The listing builds one solid part. Answer for the finished solid, in the listing's coordinates (mm). A direction names the side the tool comes from. Round coordinates to 2 decimals unless told otherwise and drop trailing zeros. Order: outer loops, then holes, each group sorted by start corner. A loop starts at its lowest first (then second) coordinate and runs counter-clockwise, first axis right, second up. Notation, with made-up numbers: (-38.75, 38.5) - (-17.75, 38.5) arc R25 ccw to (-17.75, 57.5) - close; hole circle Ø3 at (75.5, 32). An arc over 180 degrees is marked (long way). One line per item, written item: value. Start each with the question number.
1. Section A-A, the plane x = -40 is taken. Give the vertices of the cut face in (y, z), then the cut area to 3 significant figures.
2. A tool of negligible diameter and unlimited length cuts with its end or side. For faces 1 (the flat face through (-18, 0, -4.318)), 2 (the cylindrical face through (-5.586, 5.253, -2.129)), 3 (the cylindrical face through (-41.083, 13.974, 15.083)), from which of +Z, -Z, +X, -X, +Y, -Y can it reach the whole face along a straight path? Write none if from no direction.
3. Section B-B, the plane y = -26 is taken. Give the vertices of the cut face in (x, z).
4. Flat-ended cylindrical pins translate along their axes: P1, Ø3, axis at x = -9.5, y = 11, coming from the +Z side; P2, Ø12, axis at x = -41.5, z = 6, coming from the -Y side; P3, Ø2, axis at x = -35.5, z = 10, coming from the +Y side. Find the tip coordinate at first contact, or state that the pin passes through.
5. Section C-C, the plane z = 9.5 is taken. Give the vertices of the cut face in (x, y), then the cut area to 3 significant figures.
6. Section D-D, the plane x = -20.5 is taken. Give the vertices of the cut face in (y, z), then the cut area to 3 significant figures.
7. Straight lines are drawn through the part: line 1 (Z direction, x = -33, y = 7); line 2 (Z direction, x = -52, y = -16.5); line 3 (Y direction, x = -19, z = -3). For each, find the intervals that lie inside material, in ascending order.
from build123d import *

# Parameters (mm, degrees)
F0_R     = 43.938872
F1_DEPTH = 12.954
F2_R     = 13.186842
F3_DEPTH = 4.318
F4_R     = 13.716315
F5_DEPTH = 4.318


with BuildPart() as f1:
    # F0 (on Top) → F1 (new body)
    with BuildSketch(Plane.XY):
        with Locations((-21.176565, 11.984369)):
            Circle(F0_R)
    extrude(amount=F1_DEPTH)

    # F2 (on face) → F3 (join)
    with BuildSketch(Plane.XY.offset(12.954)):
        with Locations((-27.908787, 13.394361)):
            Circle(F2_R)
    extrude(amount=F3_DEPTH)

    # F4 (on face) → F5 (join)
    with BuildSketch(Plane(origin=(0, 0, 0), x_dir=(1, 0, 0), z_dir=(0, 0, -1))):
        with Locations((-18.256115, 0)):
            Circle(F4_R)
    extrude(amount=F5_DEPTH)


solid = f1.part
Answer list:
1. outline: (-27.72, 0) - (51.69, 0) - (51.69, 12.95) - (18.66, 12.95) - (18.66, 17.27) - (8.13, 17.27) - (8.13, 12.95) - (-27.72, 12.95) - close
1. area: 1,070 mm²
2. face 1: -Z, +X, -X, +Y, -Y
2. face 2: -Z
2. face 3: +Z
3. outline: (-43.26, 0) - (0.91, 0) - (0.91, 12.95) - (-43.26, 12.95) - close
4. P1: stops at z = 12.95
4. P2: stops at y = -29.55
4. P3: stops at y = 53.85
5. outline: circle Ø87.88 at (-21.18, 11.98)
5. area: 6,070 mm²
6. outline: (-31.95, 0) - (-13.53, 0) - (-13.53, -4.32) - (13.53, -4.32) - (13.53, 0) - (55.92, 0) - (55.92, 12.95) - (24.3, 12.95) - (24.3, 17.27) - (2.49, 17.27) - (2.49, 12.95) - (-31.95, 12.95) - close
6. area: 1,350 mm²
7. line 1: z = 0 to 17.27
7. line 2: z = 0 to 12.95
7. line 3: y = -13.7 to 13.7
